from build123d import *

# Parameters (mm, degrees)
BOSS_EXTRUDE3_DEPTH      = 30
BOSS_EXTRUDE3_DEPTH_BACK = 30
CUT_EXTRUDE1_DEPTH       = 9.93575
SKETCH1_R                = 1.205
CUT_EXTRUDE2_DEPTH       = 1
CUT_EXTRUDE3_REACH       = 38.571
SKETCH9_R                = 2
BOSS_EXTRUDE5_START      = -30
SKETCH20_R               = 1.7
BOSS_EXTRUDE5_DEPTH      = 15
BOSS_EXTRUDE6_START      = 30
SKETCH20_2_R             = 1.7
BOSS_EXTRUDE6_DEPTH      = 15
CUT_EXTRUDE6_START       = -30
SKETCH22_R               = 1.7
CUT_EXTRUDE6_DEPTH       = 10
CUT_EXTRUDE6_DEPTH_BACK  = 1
CUT_EXTRUDE7_START       = 30
SKETCH22_2_R             = 1.7
CUT_EXTRUDE7_DEPTH       = 10
CUT_EXTRUDE7_DEPTH_BACK  = 10


with BuildPart() as part:
    # Sketch5 → Boss-Extrude3 (new body, two sides)
    with BuildSketch(Plane.XY) as boss_extrude3_sk:
        with BuildLine():
            Line((-5.575, 9.935749893), (-18.505577921, 9.935749893))
            ThreePointArc((-18.505577921, 9.935749893), (-19.335599809, 9.493480712), (-19.431435495, 8.557877225))
            Line((-19.431435495, 8.557877225), (-15.376331952, -1.377872669))
            ThreePointArc((-15.376331952, -1.377872669), (-15.008205197, -1.830021888), (-14.450474378, -2))
            Line((-14.450474378, -2), (14.450474378, -2))
            ThreePointArc((14.450474378, -2), (15.008205197, -1.830021888), (15.376331952, -1.377872669))
            Line((15.376331952, -1.377872669), (19.431435495, 8.557877225))
            ThreePointArc((19.431435495, 8.557877225), (19.335599809, 9.493480712), (18.505577921, 9.935749893))
            Line((18.505577921, 9.935749893), (5.575, 9.935749893))
            ThreePointArc((5.575, 9.935749893), (0, 4.360749893), (-5.575, 9.935749893))
        make_face()
    extrude(amount=BOSS_EXTRUDE3_DEPTH)
    extrude(boss_extrude3_sk.sketch, amount=-BOSS_EXTRUDE3_DEPTH_BACK)

    # Sketch8 → Cut-Extrude1 (cut)
    with BuildSketch(Plane(origin=(0, 0, 0), x_dir=(1, 0, 0), z_dir=(0, 1, 0))):
        with BuildLine():
            Line((-12.5, 15), (12.5, 15))
            ThreePointArc((12.5, 15), (13.207106781, 14.707106781), (13.5, 14))
            Line((13.5, 14), (13.5, -14))
            ThreePointArc((13.5, -14), (13.207106781, -14.707106781), (12.5, -15))
            Line((12.5, -15), (-12.5, -15))
            ThreePointArc((-12.5, -15), (-13.207106781, -14.707106781), (-13.5, -14))
            Line((-13.5, -14), (-13.5, 14))
            ThreePointArc((-13.5, 14), (-13.207106781, 14.707106781), (-12.5, 15))
        make_face()
    extrude(amount=CUT_EXTRUDE1_DEPTH, mode=Mode.SUBTRACT)

    # Sketch1 → Cut-Extrude2 (cut)
    with BuildSketch(Plane(origin=(0, 0, 0), x_dir=(1, 0, 0), z_dir=(0, 1, 0))):
        with Locations((-10.105, 11.46)):
            Circle(SKETCH1_R)
        with Locations((-10.105, -11.46)):
            Circle(SKETCH1_R)
        with Locations((10.026555832, -11.46)):
            Circle(SKETCH1_R)
        with Locations((10.105, 11.46)):
            Circle(SKETCH1_R)
    extrude(amount=-CUT_EXTRUDE2_DEPTH, mode=Mode.SUBTRACT)

    # Cut-Extrude3: up to this face of the body (flat: up to its plane)
    cut_extrude3_end = Plane(part.part.faces().sort_by_distance((13.5, 4.967875, 0))[0])
    # Sketch9 → Cut-Extrude3 (cut, up to the picked face)
    with BuildSketch(Plane(origin=(13.662837448, -5.576249517, 0), x_dir=(0, 0, -1), z_dir=(0.925857573, -0.377872669, 0)), mode=Mode.PRIVATE) as cut_extrude3_sk1:
        with Locations((-9, 9.618413932)):
            Circle(SKETCH9_R)
    cut_extrude3_tool1 = split(extrude(cut_extrude3_sk1.sketch, amount=-CUT_EXTRUDE3_REACH, mode=Mode.PRIVATE), bisect_by=cut_extrude3_end, keep=Keep.BOTH, mode=Mode.PRIVATE)
    add(cut_extrude3_tool1.solids().sort_by_distance((17.297373, 3.329032, 9))[0], mode=Mode.SUBTRACT)
    # Sketch9 → Cut-Extrude3 (cut, up to the picked face)
    with BuildSketch(Plane(origin=(13.662837448, -5.576249517, 0), x_dir=(0, 0, -1), z_dir=(0.925857573, -0.377872669, 0)), mode=Mode.PRIVATE) as cut_extrude3_sk2:
        with Locations((-3, 9.618413932)):
            Circle(SKETCH9_R)
    cut_extrude3_tool2 = split(extrude(cut_extrude3_sk2.sketch, amount=-CUT_EXTRUDE3_REACH, mode=Mode.PRIVATE), bisect_by=cut_extrude3_end, keep=Keep.BOTH, mode=Mode.PRIVATE)
    add(cut_extrude3_tool2.solids().sort_by_distance((17.297373, 3.329032, 3))[0], mode=Mode.SUBTRACT)
    # Sketch9 → Cut-Extrude3 (cut, up to the picked face)
    with BuildSketch(Plane(origin=(13.662837448, -5.576249517, 0), x_dir=(0, 0, -1), z_dir=(0.925857573, -0.377872669, 0)), mode=Mode.PRIVATE) as cut_extrude3_sk3:
        with Locations((3, 9.618413932)):
            Circle(SKETCH9_R)
    cut_extrude3_tool3 = split(extrude(cut_extrude3_sk3.sketch, amount=-CUT_EXTRUDE3_REACH, mode=Mode.PRIVATE), bisect_by=cut_extrude3_end, keep=Keep.BOTH, mode=Mode.PRIVATE)
    add(cut_extrude3_tool3.solids().sort_by_distance((17.297373, 3.329032, -3))[0], mode=Mode.SUBTRACT)
    # Sketch9 → Cut-Extrude3 (cut, up to the picked face)
    with BuildSketch(Plane(origin=(13.662837448, -5.576249517, 0), x_dir=(0, 0, -1), z_dir=(0.925857573, -0.377872669, 0)), mode=Mode.PRIVATE) as cut_extrude3_sk4:
        with Locations((9, 9.618413932)):
            Circle(SKETCH9_R)
    cut_extrude3_tool4 = split(extrude(cut_extrude3_sk4.sketch, amount=-CUT_EXTRUDE3_REACH, mode=Mode.PRIVATE), bisect_by=cut_extrude3_end, keep=Keep.BOTH, mode=Mode.PRIVATE)
    add(cut_extrude3_tool4.solids().sort_by_distance((17.297373, 3.329032, -9))[0], mode=Mode.SUBTRACT)

    # Sketch20 → Boss-Extrude5 (add)
    with BuildSketch(Plane.XY.offset(BOSS_EXTRUDE5_START)):
        with BuildLine():
            Line((19.431435495, 8.557877225), (15.376331952, -1.377872669))
            ThreePointArc((15.376331952, -1.377872669), (15.008205197, -1.830021888), (14.450474378, -2))
            Line((14.450474378, -2), (24.171191968, -2))
            ThreePointArc((24.171191968, -2), (24.728922787, -1.830021888), (25.097049542, -1.377872669))
            Line((25.097049542, -1.377872669), (29.71812802, 9.944619967))
            ThreePointArc((29.71812802, 9.944619967), (27.252195948, 15.811406056), (21.385409859, 13.345473984))
            Line((21.385409859, 13.345473984), (19.431435495, 8.557877225))
        make_face()
        with Locations((25.55176894, 11.645046975)):
            Circle(SKETCH20_R, mode=Mode.SUBTRACT)
    extrude(amount=BOSS_EXTRUDE5_DEPTH)

    # Sketch20<2> → Boss-Extrude6 (add)
    with BuildSketch(Plane.XY.offset(BOSS_EXTRUDE6_START)):
        with BuildLine():
            Line((19.431435495, 8.557877225), (15.376331952, -1.377872669))
            ThreePointArc((15.376331952, -1.377872669), (15.008205197, -1.830021888), (14.450474378, -2))
            Line((14.450474378, -2), (24.171191968, -2))
            ThreePointArc((24.171191968, -2), (24.728922787, -1.830021888), (25.097049542, -1.377872669))
            Line((25.097049542, -1.377872669), (29.71812802, 9.944619967))
            ThreePointArc((29.71812802, 9.944619967), (27.252195948, 15.811406056), (21.385409859, 13.345473984))
            Line((21.385409859, 13.345473984), (19.431435495, 8.557877225))
        make_face()
        with Locations((25.55176894, 11.645046975)):
            Circle(SKETCH20_2_R, mode=Mode.SUBTRACT)
    extrude(amount=-BOSS_EXTRUDE6_DEPTH)

    # Sketch22 → Cut-Extrude6 (cut, two sides)
    with BuildSketch(Plane.XY.offset(CUT_EXTRUDE6_START)) as cut_extrude6_sk:
        with Locations((-11.667770039, 5.055979667)):
            Circle(SKETCH22_R)
    extrude(amount=CUT_EXTRUDE6_DEPTH, mode=Mode.SUBTRACT)
    extrude(cut_extrude6_sk.sketch, amount=-CUT_EXTRUDE6_DEPTH_BACK, mode=Mode.SUBTRACT)

    # Sketch22<2> → Cut-Extrude7 (cut, two sides)
    with BuildSketch(Plane.XY.offset(CUT_EXTRUDE7_START)) as cut_extrude7_sk:
        with Locations((-11.667770039, 5.055979667)):
            Circle(SKETCH22_2_R)
    extrude(amount=CUT_EXTRUDE7_DEPTH, mode=Mode.SUBTRACT)
    extrude(cut_extrude7_sk.sketch, amount=-CUT_EXTRUDE7_DEPTH_BACK, mode=Mode.SUBTRACT)


solid = part.part
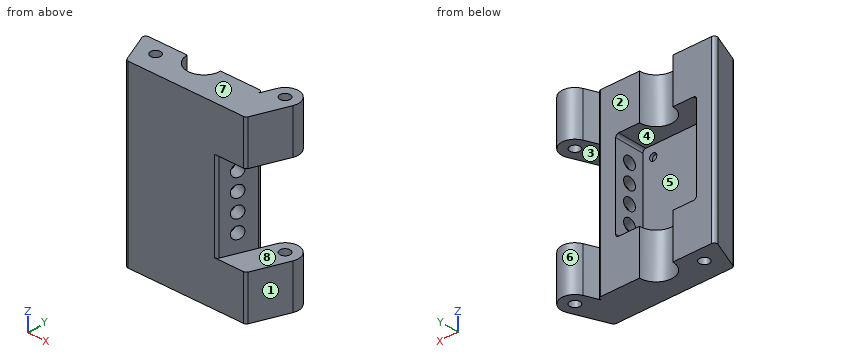
Source: CAD feature listing. Evaluate the final solid. Frame: model axes, mm. Face numbers are marked on the shaded views. A direction names the side the tool comes from. Give positions to 0.01 mm unless a question says otherwise; leave off trailing zeros. Write each loop counter-clockwise with the first axis right and the second up, starting at its lowest first coordinate (ties: lowest second). Pieces come first, ordered by that corner, then holes. Notation, with made-up numbers: M 50,-9 L 102,-9 A18 ccw 102,21 Z; hole C 50.25,8.5 d2. An arc over 180 degrees is marked long. Return JSON: item names as keys, results as strings. Group by question number.
1) Cut plane A-A, the plane x = 7. Output: boundary loops of the cut face in (y, z).
2) Pull-direction query (Z, two-part tool) for the marked faces 5, 6, 7 and 8; classes: pulls with the +Z half, pulls with the -Z half, needs draft (parallel to the pull), parting line crosses it, or undercut.
3) Cut plane D-D, the plane x = 0. Output: boundary loops of the cut face in (y, z), plus the area to 3 significant figures.
4) Cut plane B-B, the plane y = 11. Output: boundary loops of the cut face in (x, z), plus the area to 3 significant figures.
5) Material intervals for line 1 along Z through (x, y) = (6, 9); line 2 along Z through (x, y) = (14.5, 3); line 3 along X through (y, z) = (-0.35, -11.46), sorted ascending. Write a range as [from, to].
6) Cut plane C-C, the plane y = 14.75. Output: boundary loops of the cut face in (x, z).
7) Set-up query: the marked faces 1, 2, 3 and 4. Return all of +Z, -Z, +X, -X, +Y, -Y with unobstructed straight access to the full face (end or side cutting, diameter ignored); none if empty.
8) Pin query (flat end, axial travel): P1, Ø4, axis at x = 10.03, z = 11.46, coming from the +Y side; P2, Ø1, axis at x = -12, y = 5, coming from the -Z side; P3, Ø4, axis at y = 5.5, z = 2.5, coming from the +X side. Return the tip coordinate at first contact, or that it passes through.
Recorded:
{
 "1": {"outline": "M -2,-30 L 9.94,-30 L 9.94,-15 L 0,-15 L 0,15 L 9.94,15 L 9.94,30 L -2,30 Z"},
 "2": {"face 5": "undercut", "face 6": "needs draft", "face 7": "pulls with the +Z half", "face 8": "undercut"},
 "3": {"outline": "M -2,-30 L 4.36,-30 L 4.36,-15 L 0,-15 L 0,15 L 4.36,15 L 4.36,30 L -2,30 Z", "area": "251 mm²"},
 "4": {"outline": "M 20.43,-30 L 23.98,-30 L 23.98,-15 L 20.43,-15 Z; M 20.43,15 L 23.98,15 L 23.98,30 L 20.43,30 Z; M 27.12,-30 L 30.01,-30 L 30.01,-15 L 27.12,-15 Z; M 27.12,15 L 30.01,15 L 30.01,30 L 27.12,30 Z", "area": "193 mm²"},
 "5": {"line 1": "z = [-30, -15], [15, 30]", "line 2": "z = [-30, -10.46], [-7.54, -4.46], [-1.54, 1.54], [4.46, 7.54], [10.46, 30]", "line 3": "x = [-15.8, -11.31], [-8.9, 8.9], [11.31, 15.8]"},
 "6": {"outline": "M 22.29,-30 L 28.81,-30 L 28.81,-15 L 22.29,-15 Z; M 22.29,15 L 28.81,15 L 28.81,30 L 22.29,30 Z"},
 "7": {"face 1": "+Z, -Z, +X, -Y", "face 2": "+Z, -Z, -X, +Y", "face 3": "+X, -Y", "face 4": "+Y"},
 "8": {"P1": "stops at y = 0", "P2": "stops at z = -20", "P3": "stops at x = 19"}
}
